Autodesk Inventor part; units mm, degrees
ref_plane "YZ Plane" through (0, 0, 0) normal (1, 0, 0) x (0, 1, 0)
ref_plane "XZ Plane" through (0, 0, 0) normal (0, 1, 0) x (-1, 0, 0)
ref_plane "XY Plane" through (0, 0, 0) normal (0, 0, 1) x (1, 0, 0)
ref_plane "Work Plane1" through (0, 0, 0) normal (0, 0, 1) x (1, 0, 0)
sketch "Sketch1" plane through (0, 0, 0) normal (0, 0, 1) x (1, 0, 0)
  line L0 (55, -528.7123) -> (55, -461.767)
  line L1 (55, -461.767) -> (20, -461.767)
  line L2 (20, -461.767) -> (20, -528.7123)
  arc A0 (20, -528.7123) -> (55, -528.7123) centre (37.5, -528.7123) ccw
  line L3 (43.5, -461.767) -> (31.5, -461.767)
  line L4 (37.5, -461.767) -> (37.5, -485.2876) construction
  arc A1 (30.6824, -513.1447) -> (23.108, -519.6737) centre (26.8952, -516.4092) ccw
  line L5 (88.3973, -595.4186) -> (23.108, -519.6737)
  line L6 (30.6824, -513.1447) -> (95.9718, -588.8897)
  arc A2 (88.3973, -595.4186) -> (95.9718, -588.8897) centre (92.1846, -592.1541) ccw
  line L7 (92.1846, -592.1541) -> (26.8952, -516.4092) construction
  circle A3 centre (37.5, -528.7123) radius 5
  point P0 (0, 0)
  dimension "d0" = 23.5206
  dimension "d1" = 35
extrude "Extrusion1" add sketch "Sketch1" along normal mid plane 40 contours A0 L6 A1 L5 L2 L1 L0 | A0 L5 A3 L6 | A3 L5 A1 L6
sketch "Sketch2" plane through (20, -528.7123, 20) normal (-1, 0, 0) x (0, 0, 1)
  line L0 (-11, 54.2123) -> (-29, 54.2123)
  line L1 (-11, 61.2123) -> (-29, 61.2123)
  line L2 (-34.8412, -128.9954) -> (-34.8412, 22.4945)
  line L3 (-4.8412, 22.4945) -> (-4.8412, -128.9954)
  line L4 (-40, -17.5) -> (0, -17.5)
  line L5 (-4.8412, -17.5) -> (-4.8412, 61.2123)
  line L6 (-4.8412, 61.2123) -> (-34.8412, 61.2123)
  line L7 (-34.8412, 61.2123) -> (-34.8412, -17.5)
  point P0 (-20, 528.7123)
  point P1 (-34.8412, 22.4945)
  point P2 (-29, 61.2123)
extrude "Extrusion2" cut sketch "Sketch2" against normal through all
sketch "Sketch3" plane through (20, -467.5, -14.8412) normal (0, -1, 0) x (1, 0, 0)
  circle A0 centre (17.5, 14.8412) radius 6
  point P0 (-20, 14.8412)
extrude "Extrusion3" cut sketch "Sketch3" against normal through all
properties part number "Junta Revoluta"
Input: part model. Units: mm. Frame: model coordinates. A direction names the side the tool comes from. Give positions to 0.01 mm unless a question says otherwise; leave off trailing zeros. Order: outer loops, then holes, each group sorted by start corner. A loop starts at its lowest first (then second) coordinate and runs counter-clockwise, first axis right, second up. Notation, with made-up numbers: M 69,48.5 L 73,48.5 A18 cw 73,59.5 Z; hole C 31.25,19 d7. An arc over 180 degrees is marked long. Return JSON: item names as keys, results as strings.
1) Section query D-D on z = -17. Output: boundary loops of the cut face in (x, y).
Taken from the geometry:
{"outline": "M 20,-528.71 A17.5 ccw 55,-528.71 L 55,-461.77 L 20,-461.77 Z; hole C 37.5,-528.71 d10"}
2) Section query B-B on y = -521.5. Output: boundary loops of the cut face in (x, z), and give its area (3 significant figures).
Taken from the geometry:
{"outline": "M 20,-20 L 55,-20 L 55,-14.84 L 20,-14.84 Z; M 20,15.16 L 55,15.16 L 55,20 L 20,20 Z", "area": "350 mm2"}
3) Contact query for flat-ended pins moving along their axis: pin 1 (15 mm diameter, centred on x = 42.5, z = -6.5, fed in from -Y); pin 2 (11.5 mm diameter, centred on x = 37.5, y = -528.71, fed in from +Z). Output: stop coordinate, or through.
Taken from the geometry:
{"pin 1": "stops at y = -467.5", "pin 2": "stops at z = 20"}
4) Access query for faces 4 (the face through (37, -507, -14.841)), 5 (the face through (37.88, -546.21, 17.55)). Directions: +Z, -Z, +X, -X, +Y, -Y. A direction counts if a zero-diameter tool reaches every point of the face in a straight line with its end or side. Return the directions, or none.
Taken from the geometry:
{"face 4": "+X, -X, -Y", "face 5": "+Z, -Z, -Y"}
5) Section query A-A on x = 37.5. Output: boundary loops of the cut face in (y, z).
Taken from the geometry:
{"outline": "M -546.21,-20 L -533.71,-20 L -533.71,-14.84 L -546.21,-14.84 Z; M -546.21,15.16 L -533.71,15.16 L -533.71,20 L -546.21,20 Z; M -523.71,-20 L -461.77,-20 L -461.77,-6 L -467.5,-6 L -467.5,-14.84 L -523.71,-14.84 Z; M -523.71,15.16 L -467.5,15.16 L -467.5,6 L -461.77,6 L -461.77,20 L -523.71,20 Z"}
6) Line query: L1, parallel to Z at x = 33, y = -472; L2, parallel to Y at x = 37.5, z = 17.9; L3, parallel to Y at x = 51.5, z = 12.5. Output: solid intervals per line, ascending. Write a range as [from, to].
Taken from the geometry:
{"L1": "z = [-20, -14.84], [15.16, 20]", "L2": "y = [-546.21, -533.71], [-523.71, -461.77]", "L3": "y = [-467.5, -461.77]"}
7) Mould query, pull axis X, two halves, no side actions, for faces 1 (the face through (37, -506, 15.159)), 2 (the face through (32.74, -464.67, -3.65)), 3 (the face through (20, -490, -15)). Classes: released by +X, released by -X, zero draft, split by the parting line, or undercut.
Taken from the geometry:
{"face 1": "zero draft", "face 2": "undercut", "face 3": "released by -X"}
8) Section query C-C on z = 0. Output: boundary loops of the cut face in (x, y), and give its area (3 significant figures).
Taken from the geometry:
{"outline": "M 20,-467.5 L 31.5,-467.5 L 31.5,-461.77 L 20,-461.77 Z; M 43.5,-467.5 L 55,-467.5 L 55,-461.77 L 43.5,-461.77 Z", "area": "132 mm2"}
